from build123d import *

# Parameters (mm, degrees)
SKETCH1_W = 25
SKETCH1_H = 25


with BuildPart() as part:
    # Sweep1: sweep along a path in Sketch2
    with BuildLine(Plane(origin=(0, 0, 0), x_dir=(1, 0, 0), z_dir=(0, 1, 0))) as sweep1_path:
        Line((0, 0), (0, -62))
        Line((0, -62), (298, -62))
        Line((298, -62), (298, 0))
    # Sketch1 → Sweep1 (sweep)
    with BuildSketch(Plane.XY):
        Rectangle(SKETCH1_W, SKETCH1_H)
    sweep(path=sweep1_path.line, transition=Transition.RIGHT)


solid = part.part
Input: part model. Units: mm. Frame: model coordinates. A direction names the side the tool comes from. Coordinates: 2 decimals unless noted, no trailing zeros. Loops run counter-clockwise (first coordinate to the right, second up) from the corner with the lowest first, then second, coordinate; pieces in that order, holes last.
Q1. Draft query along X for faces 1 (the face through (12.5, 0, 25)), 2 (the face through (-12.5, 0, 38)), 3 (the face through (310.5, 0, 37)). Return one class per face: +X half, -X half, draft (parallel to the pull), parting line (faces both ways), or undercut.
Q2. Material intervals for line 1 (X direction, y = -10, z = 20.5); line 2 (Z direction, x = 24.5, y = 11.75), sorted ascending.
Q3. Cut plane C-C (x = 44). Output: boundary loops of the cut face in (y, z), then the cut area to 3 significant figures.
Q4. Cut plane B-B (y = -2.25). Output: boundary loops of the cut face in (x, z).
Q5. Contact query for a flat-ended pin moving along its axis: pin 1 (4 mm diameter, centred on x = 97.5, y = 2.5, fed in from -Z). Output: stop coordinate, or through.
Q6. Cut plane A-A (z = 40). Output: boundary loops of the cut face in (x, y).
Q7. Set-up query: faces 4 (the face through (151, 0, 49.5)), 5 (the face through (147, -12.5, 54)). Return all of +Z, -Z, +X, -X, +Y, -Y with unobstructed straight access to the full face (end or side cutting, diameter ignored); none if empty.
Working result:
1. face 1: undercut
1. face 2: -X half
1. face 3: +X half
2. line 1: x = -12.5 to 12.5, 285.5 to 310.5
2. line 2: z = 49.5 to 74.5
3. outline: (-12.5, 49.5) - (12.5, 49.5) - (12.5, 74.5) - (-12.5, 74.5) - close
3. area: 625 mm2
4. outline: (-12.5, 0) - (12.5, 0) - (12.5, 49.5) - (285.5, 49.5) - (285.5, 0) - (310.5, 0) - (310.5, 74.5) - (-12.5, 74.5) - close
5. pin 1: stops at z = 49.5
6. outline: (-12.5, -12.5) - (12.5, -12.5) - (12.5, 12.5) - (-12.5, 12.5) - close; (285.5, -12.5) - (310.5, -12.5) - (310.5, 12.5) - (285.5, 12.5) - close
7. face 4: -Z, +Y, -Y
7. face 5: +Z, -Z, +X, -X, -Y
